Input: part model. Units: mm. Frame: model coordinates. Face numbers are marked on the shaded views. A direction names the side the tool comes from. Round coordinates to 2 decimals unless told otherwise and drop trailing zeros. Loops run counter-clockwise (first coordinate to the right, second up) from the corner with the lowest first, then second, coordinate; pieces in that order, holes last. Notation, with made-up numbers: (59, 6.25) -> (105, 6.25) arc R13 ccw to (105, 14.25) -> close; hole circle Ø1 at (53, 67). An arc over 180 degrees is marked (long way). Answer as a JSON object with one key per item and string values.
```python
from build123d import *

# Parameters (mm, degrees)
WYTNIJ_WYCI_GNI_CIE1_DEPTH = 22
WYTNIJ_WYCI_GNI_CIE2_DEPTH = 120
SZYK_KO_OWY2_COUNT         = 16
SFAZOWANIE1_SIZE           = 3


with BuildPart() as part:
    # Szkic1 → Obrót1 (revolve)
    with BuildSketch(Plane.XY, mode=Mode.PRIVATE) as obr_t1_sk:
        Polygon((0, 0), (0, 30), (70, 30), (70, 55), (270, 55), (270, 65), (420, 65), (420, 75), (520, 75), (520, 65), (820, 65), (820, 55), (880, 55), (880, 40), (1080, 40), (1080, 30), (1140, 30), (1140, 0), align=None)
    revolve(obr_t1_sk.sketch.rotate(Axis((0, 0, 0), (1, 0, 0)), 180), axis=Axis((0, 0, 0), (1, 0, 0)))

    # Szkic2 → Wytnij-wyciągnięcie1 (cut)
    with BuildSketch(Plane(origin=(0, -55, 0), x_dir=(-1, 0, 0), z_dir=(0, -1, 0))):
        with BuildLine():
            Line((-210, 12), (-130, 12))
            ThreePointArc((-130, 12), (-118, 0), (-130, -12))
            Line((-130, -12), (-210, -12))
            ThreePointArc((-210, -12), (-222, 0), (-210, 12))
        make_face()
    extrude(amount=-WYTNIJ_WYCI_GNI_CIE1_DEPTH, mode=Mode.SUBTRACT)

    # Szkic4 → Wytnij-wyciągnięcie2 (cut)
    with BuildSketch(Plane.ZY.offset(-270)):
        Polygon((0, -65.135380743), (0, -59.348257278), (-6, -59.348257278), (-6, -71.348257278), (0, -71.348257278), align=None)
        Polygon((6, -59.348257278), (0, -59.348257278), (0, -65.135380743), (0, -71.348257278), (6, -71.348257278), align=None)
    wytnij_wyci_gni_cie2 = extrude(amount=-WYTNIJ_WYCI_GNI_CIE2_DEPTH, mode=Mode.SUBTRACT)

    # Szyk kołowy2: Wytnij-wyciągnięcie2 ×16 about axis
    szyk_ko_owy2_axis = Axis((0, 0, 0), (1, 0, 0))
    for i in range(1, SZYK_KO_OWY2_COUNT):
        add(wytnij_wyci_gni_cie2.rotate(szyk_ko_owy2_axis, i * 360 / SZYK_KO_OWY2_COUNT), mode=Mode.SUBTRACT)

    # Sfazowanie1
    sfazowanie1_edges = [part.edges().sort_by_distance(p)[0] for p in [
        (1140, 30, 0),
        (1080, 30, 0),
        (1080, 40, 0),
        (880, 40, 0),
        (880, 55, 0),
        (820, 55, 0),
        (820, 65, 0),
        (520, 65, 0),
        (520, 75, 0),
        (420, 75, 0),
        (420, 65, 0),
        (270, -63.751043226, 12.680870931),
        (270, 55, 0),
        (70, 55, 0),
        (70, 30, 0),
        (0, 30, 0),
        (270, -54.0455248, 36.112065146),
        (270, -36.112065146, 54.0455248),
        (270, -12.680870931, 63.751043226),
        (270, 12.680870931, 63.751043226),
        (270, 36.112065146, 54.0455248),
        (270, 54.0455248, 36.112065146),
        (270, 63.751043226, 12.680870931),
        (270, 63.751043226, -12.680870931),
        (270, 54.0455248, -36.112065146),
        (270, 36.112065146, -54.0455248),
        (270, 12.680870931, -63.751043226),
        (270, -12.680870931, -63.751043226),
        (270, -36.112065146, -54.0455248),
        (270, -54.0455248, -36.112065146),
        (270, -63.751043226, -12.680870931),
    ]]
    chamfer(sfazowanie1_edges, length=SFAZOWANIE1_SIZE)


solid = part.part
```
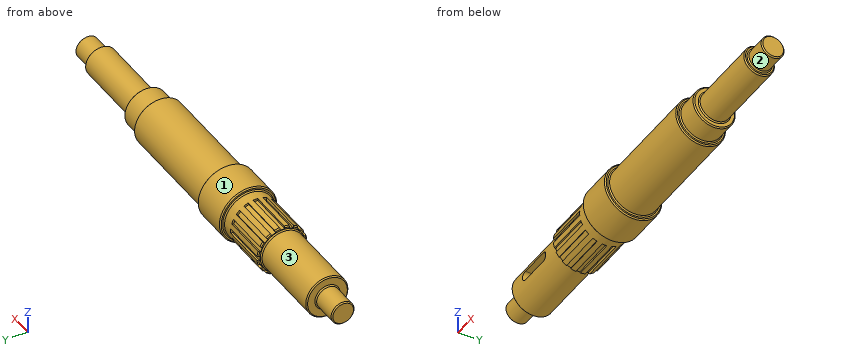
1) Section B-B, the plane x = 1013. Output: boundary loops of the cut face in (y, z), plus the area to 3 significant figures.
Output:
{"outline": "circle Ø80 at (0, 0)", "area": "5,030 mm^2"}
2) Section A-A, the plane x = 652. Output: boundary loops of the cut face in (y, z), plus the area to 3 significant figures.
Output:
{"outline": "circle Ø130 at (0, 0)", "area": "13,300 mm^2"}
3) Contact query for flat-ended pins moving along their axis: P1, Ø6, axis at x = 179, y = -45, coming from the -Z side; P2, Ø6, axis at y = 41, z = -45.5, coming from the -X side; P3, Ø3.5, axis at x = 355.5, y = 2, coming from the +Z side; P4, Ø12, axis at x = 1010.5, y = 49, coming from the +Z side. Output: stop coordinate, or through.
Output:
{"P1": "stops at z = -35.51", "P2": "stops at x = 270", "P3": "stops at z = 59.35", "P4": "passes through"}
4) Reachability of the marked faces 1, 2 and 3 from +Z, -Z, +X, -X, +Y, -Y: full face, straight path, thin tool, end or side. Return the list, or none.
Output:
{"face 1": "+X, -X", "face 2": "+X", "face 3": "-X"}
5) Ray query, probe 1 along X at (y, z) = (57, -13); probe 2 along X at (y, z) = (8, 39); probe 3 along Z at (x, y) = (234.5, -30). Return the intervals inside material, ascending.
Output:
{"probe 1": "x = 270 to 820", "probe 2": "x = 70 to 1077.19", "probe 3": "z = -46.1 to 46.1"}
